Part print with two shaded views. Sizes in mm from the minimum x, y, z corner. Give positions to 0.01 mm unless a question says otherwise; leave off trailing zeros. Order: outer loops, then holes, each group sorted by start corner. A loop starts at its lowest first (then second) coordinate and runs counter-clockwise, first axis right, second up. Notation, with made-up numbers: M -32.5,-36 L 12.5,-36 A19 ccw 12.5,-13 Z; hole C 66,-29.5 d11. An arc over 180 degrees is marked long. Answer as CSV lines item,"result".
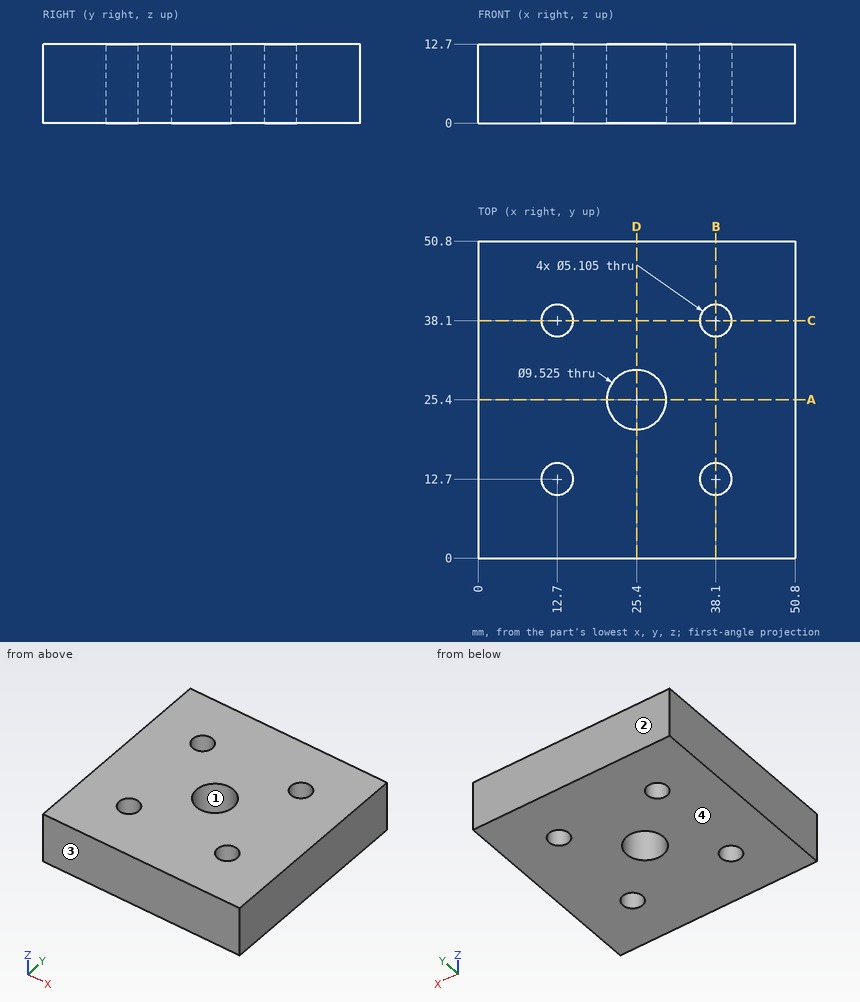
Item 1: Band-saw the part on B-B (x = 38.1). Give the cut face in (y, z).
Geometry says:
outline,"M 0,0 L 10.15,0 L 10.15,12.7 L 0,12.7 Z; M 15.25,0 L 35.55,0 L 35.55,12.7 L 15.25,12.7 Z; M 40.65,0 L 50.8,0 L 50.8,12.7 L 40.65,12.7 Z"
Item 2: Probe line 1 along Y through (x, z) = (38.1, 7); line 2 along X through (y, z) = (12.5, 5) (1 decimal). List the from-to ranges inside material, lowest first. Write a range as from..to.
Geometry says:
line 1,"y = 0..10.15, 15.25..35.55, 40.65..50.8"
line 2,"x = 0..10.2, 15.2..35.6, 40.6..50.8"
Item 3: Pull direction Y, two halves, no side cores. Call the marked faces 1, 2, 3 and 4: released by +Y, released by -Y, zero draft, split by the parting line, or undercut.
Geometry says:
face 1,"undercut"
face 2,"released by +Y"
face 3,"released by -Y"
face 4,"zero draft"
Item 4: Band-saw the part on A-A (y = 25.4). Give the cut face in (x, z).
Geometry says:
outline,"M 0,0 L 20.64,0 L 20.64,12.7 L 0,12.7 Z; M 30.16,0 L 50.8,0 L 50.8,12.7 L 30.16,12.7 Z"
Item 5: Drop a flat-ended pin along its axis: pin 1 (8 mm diameter, centred on x = 38.1, y = 38.1, fed in from +Z). Give the stop position or say it passes through.
Geometry says:
pin 1,"stops at z = 12.7"
